Autodesk Inventor part; units mm, degrees
ref_plane "YZ Plane" through (0, 0, 0) normal (1, 0, 0) x (0, 1, 0)
ref_plane "XZ Plane" through (0, 0, 0) normal (0, 1, 0) x (-1, 0, 0)
ref_plane "XY Plane" through (0, 0, 0) normal (0, 0, 1) x (1, 0, 0)
sketch "Sketch1" plane through (0, 0, 0) normal (0, 0, 1) x (1, 0, 0)
  line L0 (19.05, -19.05) -> (-19.05, -19.05)
  line L1 (-19.05, -19.05) -> (-19.05, 19.05)
  line L2 (-19.05, 19.05) -> (19.05, 19.05)
  line L3 (19.05, 19.05) -> (19.05, -19.05)
  line L4 (19.05, -19.05) -> (-19.05, 19.05) construction
  line L5 (-19.05, -19.05) -> (19.05, 19.05) construction
  line L6 (15.875, 15.875) -> (-15.875, 15.875)
  line L7 (-15.875, 15.875) -> (-15.875, -15.875)
  line L8 (-15.875, -15.875) -> (15.875, -15.875)
  line L9 (15.875, -15.875) -> (15.875, 15.875)
  point P0 (0, 0)
  dimension "d0" = 38.1
  dimension "d1" = 38.1
  dimension "d2" = 3.175
extrude "Extrusion1" add sketch "Sketch1" along normal blind 152.4
sketch "Sketch2" plane through (19.05, -19.05, 0) normal (1, 0, 0) x (0, 0, -1)
  line L0 (0, 0) -> (0, 38.1)
  line L1 (0, 38.1) -> (-152.4, 38.1)
  line L2 (-152.4, 0) -> (-152.4, 38.1)
  line L3 (0, 0) -> (-152.4, 0)
  line L4 (-76.2, 38.1) -> (-76.2, 0) construction
  line L5 (-152.4, 19.05) -> (0, 19.05) construction
  circle A0 centre (-114.3, 31.115) radius 2.0955
  circle A1 centre (-146.304, 31.115) radius 2.0955
  dimension "d5" = 4.191
  dimension "d7" = 114.3
  dimension "d8" = 4.191
  dimension "d9" = 6.985
  dimension "d10" = 6.985
  dimension "d11" = 32.004
extrude "Extrusion2" cut sketch "Sketch2" against normal through all contours A0 | A1
sketch "Sketch3" plane through (19.05, -19.05, 0) normal (1, 0, 0) x (0, 0, -1)
  line L0 (0, 38.1) -> (-152.4, 38.1) construction
  line L1 (-76.2, 38.1) -> (-76.2, 0) construction
  line L2 (0, 0) -> (-152.4, 0) construction
  line L3 (0, 19.05) -> (-152.4, 19.05) construction
  line L4 (-152.4, 38.1) -> (-152.4, 0) construction
  circle A0 centre (-6.35, 29.21) radius 2.25
  line L5 (0, 0) -> (0, 38.1)
  circle A1 centre (-6.35, 8.89) radius 2.25
  circle A2 centre (-25.4, 29.21) radius 2.25
  circle A3 centre (-25.4, 8.89) radius 2.25
  dimension "d14" = 4.5
  dimension "d15" = 6.35
  dimension "d16" = 4.5
  dimension "d17" = 6.35
  dimension "d18" = 8.89
  dimension "d19" = 8.89
  dimension "d20" = 4.5
  dimension "d21" = 19.05
  dimension "d22" = 4.5
extrude "Extrusion3" cut sketch "Sketch3" against normal through all
properties part number "CS_Climb_Outer_Tube"
Geometry: final body of the model. Coordinates: model frame, mm. A direction names the side the tool comes from. Round coordinates to 2 decimals unless told otherwise and drop trailing zeros. Write each loop counter-clockwise with the first axis right and the second up, starting at its lowest first coordinate (ties: lowest second). Pieces come first, ordered by that corner, then holes. Notation, with made-up numbers: M 86,-2.5 L 109,-2.5 A25 cw 109,9.5 Z; hole C 17,36.5 d6. An arc over 180 degrees is marked long. Answer in a Markdown table with one row per item. Add a question column.
(1) Cut plane A-A, the plane y = -10.16. Return the cut outline in (x, z) (3 decimals), then the cut area to 3 significant figures.
(2) Draft query along Z for faces 3 (the face through (0, 19.05, 75)), 4 (the face through (-17, 0, 152.4)), 5 (the face through (17.485, 12.057, 5.14)). Return one class per face: pulls with the +Z half, pulls with the -Z half, needs draft (parallel to the pull), parting line crosses it, or undercut.
(3) Ray query, L1, parallel to Y at x = -17.75, z = 6.35; L2, parallel to Y at x = -10, z = 23 (3 decimals). Return the intervals inside material, ascending.
(4) Cut plane B-B, the plane x = 12. Return the cut outline in (y, z) (3 decimals), then the cut area to 3 significant figures.
(5) Reachability of faces 1 (the face through (-17, 0, 0)), 2 (the face through (0, 15.875, 75)) from +Z, -Z, +X, -X, +Y, -Y: full face, straight path, thin tool, end or side. Return the list, or none.
(6) Contact query for a flat-ended pin moving along its axis: pin 1 (6.5 mm diameter, centred on y = 12.065, z = 114.3, fed in from +X). Output: stop coordinate, or through.
Established:
| question | item | result |
|---|---|---|
| 1 | outline | M -19.05,0 L -15.875,0 L -15.875,4.1 L -19.05,4.1 Z; M -19.05,8.6 L -15.875,8.6 L -15.875,23.15 L -19.05,23.15 Z; M -19.05,27.65 L -15.875,27.65 L -15.875,152.4 L -19.05,152.4 Z; M 15.875,0 L 19.05,0 L 19.05,4.1 L 15.875,4.1 Z; M 15.875,8.6 L 19.05,8.6 L 19.05,23.15 L 15.875,23.15 Z; M 15.875,27.65 L 19.05,27.65 L 19.05,152.4 L 15.875,152.4 Z |
| 1 | area | 911 mm² |
| 2 | face 3 | needs draft |
| 2 | face 4 | pulls with the +Z half |
| 2 | face 5 | undercut |
| 3 | L1 | -19.05 to -12.41, -7.91 to 7.91, 12.41 to 19.05 |
| 3 | L2 | -19.05 to -15.875, 15.875 to 19.05 |
| 4 | outline | M -19.05,0 L -15.875,0 L -15.875,152.4 L -19.05,152.4 Z; M 15.875,0 L 19.05,0 L 19.05,152.4 L 15.875,152.4 Z |
| 4 | area | 968 mm² |
| 5 | face 1 | -Z, +X, -X, +Y, -Y |
| 5 | face 2 | +Z, -Z |
| 6 | pin 1 | x = 19.05 |
